Solid Edge part; units mm, degrees
sketch "Sketch1" plane through (0, 0, 0) normal (0, 0, 1) x (1, 0, 0)
  line L0 (-3.47, -6) -> (3.47, -6)
  line L1 (3.47, -6) -> (3.47, 6)
  line L2 (3.47, 6) -> (-3.47, 6)
  line L3 (-3.47, 6) -> (-3.47, -6)
  dimension "D1" = 3.47
  dimension "D2" = 3.47
extrude "Protrusion1" add sketch "Sketch1" against normal blind 0.41
sketch "Sketch2" plane through (0, 0, 0) normal (0, 0, 1) x (1, 0, 0)
  circle A0 centre (-2.96, 3) radius 0.5
  circle A1 centre (-2.96, 0) radius 0.5
  circle A2 centre (-2.96, -3) radius 0.5
extrude "Extrusionsausschnitt_1" cut sketch "Sketch2" against normal blind 0.01
mirror "Mirror1" about plane through (0, 0, 0) normal (1, 0, 0) of "Extrusionsausschnitt_1"
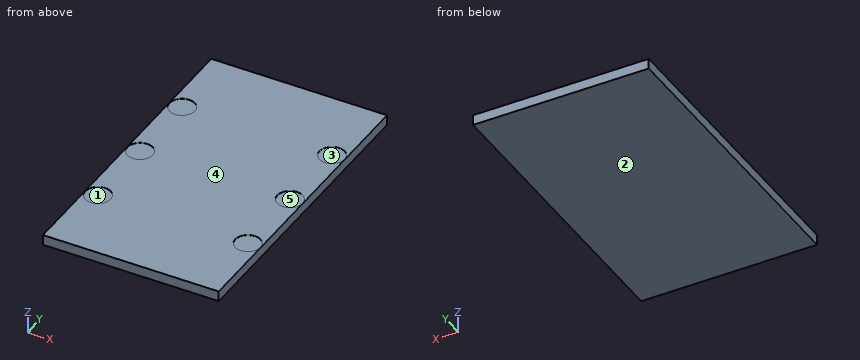
Work out the finished part from the listing and answer in its coordinate system (mm). Face numbers are marked on the shaded views. A direction names the side the tool comes from. Round coordinates to 2 decimals unless told otherwise and drop trailing zeros.
1) Determine the mould class of the marked faces 1, 2 and 3 for opening direction Y: pulls with the +Y half, pulls with the -Y half, needs draft (parallel to the pull), parting line crosses it, or undercut.
2) A flat-ended cylindrical pin translates along its axis: P1, Ø0.5, axis at x = -3, y = -3, coming from the +Z side. Find the tip coordinate at first contact, or state that the pin passes through.
3) Consider probe 1 along Z at (x, y) = (3.25, -3). Determine where the line is inside the solid, lowest interval first.
4) Which of the six approach directions +Z, -Z, +X, -X, +Y, -Y give full straight-line access (tool end or side, diameter ignored) to the marked faces 4 and 5?
Entries:
1. face 1: undercut
1. face 2: needs draft
1. face 3: undercut
2. P1: stops at z = -0.01
3. probe 1: z = -0.41 to -0.01
4. face 4: +Z, +X, -X, +Y, -Y
4. face 5: +Z
